from build123d import *

# Parameters (mm, degrees)
ESQUISSE1_R                  = 23
BOSS_EXTRU_1_DEPTH           = 6
ESQUISSE2_R                  = 12.5
BOSS_EXTRU_2_DEPTH           = 10
ESQUISSE3_R                  = 3.25
ENL_V_MAT_EXTRU_1_DEPTH      = 16
ENL_V_MAT_EXTRU_2_REACH      = 38.249
ENL_V_MAT_EXTRU_2_END_RADIUS = 12.5
ESQUISSE4_R                  = 2.5
ESQUISSE5_R                  = 2.75
ENL_V_MAT_EXTRU_3_DEPTH      = 6
R_P_T_PAR_COURBE1_COUNT      = 3
ENL_V_MAT_EXTRU_4_REACH      = 38.249
ESQUISSE6_W                  = 8
ESQUISSE6_H                  = 4


with BuildPart() as part:
    # Esquisse1 → Boss.-Extru.1 (new body)
    with BuildSketch(Plane.XY):
        Circle(ESQUISSE1_R)
    extrude(amount=BOSS_EXTRU_1_DEPTH)

    # Esquisse2 → Boss.-Extru.2 (add)
    with BuildSketch(Plane.XY.offset(6)):
        Circle(ESQUISSE2_R)
    extrude(amount=BOSS_EXTRU_2_DEPTH)

    # Esquisse3 → Enlèv. mat.-Extru.1 (cut)
    with BuildSketch(Plane.XY.offset(16)):
        Circle(ESQUISSE3_R)
    extrude(amount=-ENL_V_MAT_EXTRU_1_DEPTH, mode=Mode.SUBTRACT)

    # Enlèv. mat.-Extru.2: up to this cylinder (the profile starts inside it)
    enl_v_mat_extru_2_end = Plane(origin=(0, 0, 11), z_dir=(0, 0, -1)) * Cylinder(ENL_V_MAT_EXTRU_2_END_RADIUS, 102.498, mode=Mode.PRIVATE)
    # Esquisse4 → Enlèv. mat.-Extru.2 (cut, up to the surface)
    with BuildSketch(Plane(origin=(0, 0, 0), x_dir=(1, 0, 0), z_dir=(0, 1, 0)), mode=Mode.PRIVATE) as enl_v_mat_extru_2_sk1:
        with Locations(Location((0, -11, 0), (0, 0, 270))):
            Circle(ESQUISSE4_R)
    enl_v_mat_extru_2_tool1 = extrude(enl_v_mat_extru_2_sk1.sketch, amount=-ENL_V_MAT_EXTRU_2_REACH, mode=Mode.PRIVATE) & enl_v_mat_extru_2_end
    add(enl_v_mat_extru_2_tool1.solids().sort_by_distance((0, 0, 11))[0], mode=Mode.SUBTRACT)

    # Esquisse5 → Enlèv. mat.-Extru.3 (cut)
    with BuildSketch(Plane.XY.offset(6)):
        with Locations((0, 18)):
            Circle(ESQUISSE5_R)
    enl_v_mat_extru_3 = extrude(amount=-ENL_V_MAT_EXTRU_3_DEPTH, mode=Mode.SUBTRACT)

    # Répét. par courbe1: Enlèv. mat.-Extru.3 ×3 about axis
    r_p_t_par_courbe1_axis = Axis((0, 0, 6), (0, 0, -1))
    for i in range(1, R_P_T_PAR_COURBE1_COUNT):
        add(enl_v_mat_extru_3.rotate(r_p_t_par_courbe1_axis, i * 360 / R_P_T_PAR_COURBE1_COUNT), mode=Mode.SUBTRACT)

    # Enlèv. mat.-Extru.4: up to this face of the body (flat: up to its plane)
    enl_v_mat_extru_4_end = Plane(part.part.faces().sort_by_distance((-22.349461761, 0, 6))[0])
    # Esquisse6 → Enlèv. mat.-Extru.4 (cut, up to the picked face)
    with BuildSketch(Plane.XY.offset(16), mode=Mode.PRIVATE) as enl_v_mat_extru_4_sk1:
        with Locations((0, -7)):
            Rectangle(ESQUISSE6_W, ESQUISSE6_H)
    enl_v_mat_extru_4_tool1 = split(extrude(enl_v_mat_extru_4_sk1.sketch, amount=-ENL_V_MAT_EXTRU_4_REACH, mode=Mode.PRIVATE), bisect_by=enl_v_mat_extru_4_end, keep=Keep.BOTH, mode=Mode.PRIVATE)
    add(enl_v_mat_extru_4_tool1.solids().sort_by(Axis((0, -7, 16), (0, 0, -1)))[0], mode=Mode.SUBTRACT)


solid = part.part
Part model, mm, in its own coordinate system. A direction names the side the tool comes from. Give positions to 0.01 mm unless a question says otherwise; leave off trailing zeros. Loops run counter-clockwise (first coordinate to the right, second up) from the corner with the lowest first, then second, coordinate; pieces in that order, holes last.
(1) Band-saw the part on D-D (y = -4). Write the cut outline in (x, z).
Return value:
outline: (-22.65, 0) - (22.65, 0) - (22.65, 6) - (11.84, 6) - (11.84, 16) - (-11.84, 16) - (-11.84, 6) - (-22.65, 6) - close; hole circle Ø5 at (0, 11)
(2) Pull direction Y, two halves, no side cores. Call faces 1 (the cylindrical face through (11.923, 3.755, 10.93)), 2 (the flat face through (3, 3, 16)), 3 (the cylindrical face through (18.13, -10.05, 3.04)): pulls with the +Y half, pulls with the -Y half, needs draft (parallel to the pull), parting line crosses it, or undercut.
Return value:
face 1: parting line crosses it
face 2: needs draft
face 3: undercut
(3) Band-saw the part on A-A (x = 0). Write the cut outline in (y, z), and give its area (3 significant figures).
Return value:
outline: (-23, 0) - (-3.25, 0) - (-3.25, 8.5) - (-5, 8.5) - (-5, 6) - (-9, 6) - (-9, 8.5) - (-12.5, 8.5) - (-12.5, 6) - (-23, 6) - close; (-12.5, 13.5) - (-9, 13.5) - (-9, 16) - (-12.5, 16) - close; (-5, 13.5) - (-3.25, 13.5) - (-3.25, 16) - (-5, 16) - close; (3.25, 0) - (15.25, 0) - (15.25, 6) - (12.5, 6) - (12.5, 16) - (3.25, 16) - close; (20.75, 0) - (23, 0) - (23, 6) - (20.75, 6) - close
area: 323 mm2
(4) Pin check, flat tips, straight feed: pin 1 (4 mm diameter, centred on y = 6, z = 4.5, fed in from -X); pin 2 (2 mm diameter, centred on x = 0.5, y = -7, fed in from +Z); pin 3 (8 mm diameter, centred on x = 8, z = 10.5, fed in from -Y). Stop position of each tip, or through.
Return value:
pin 1: stops at x = -22.65
pin 2: stops at z = 6
pin 3: stops at y = -11.84
(5) Band-saw the part on B-B (y = 18). Write the cut outline in (x, z).
Return value:
outline: (-14.32, 0) - (-2.75, 0) - (-2.75, 6) - (-14.32, 6) - close; (2.75, 0) - (14.32, 0) - (14.32, 6) - (2.75, 6) - close
(6) Band-saw the part on C-C (x = -15.5). Write the cut outline in (y, z), and give its area (3 significant figures).
Return value:
outline: (-16.99, 0) - (-11.75, 0) - (-11.75, 6) - (-16.99, 6) - close; (-6.25, 0) - (16.99, 0) - (16.99, 6) - (-6.25, 6) - close
area: 171 mm2
(7) Drill centre lines: line 1 along Y through (x, z) = (0, 2.6); line 2 along Z through (x, y) = (0, -4.15); line 3 along Z through (x, y) = (11, -16.5). Where is each one in solid material? Low to high.
Return value:
line 1: y = -23 to -3.25, 3.25 to 15.25, 20.75 to 23
line 2: z = 0 to 8.5, 13.5 to 16
line 3: z = 0 to 6
(8) 3-axis set-ups, long thin cutter, end or side, ignore diameter. For faces 4 (the cylindrical face through (-0.423, 3.222, 8.112)), 5 (the cylindrical face through (0.751, -3.843, 13.385)), 6 (the flat face through (-4, -7, 11)): which of +Z, -Z, +X, -X, +Y, -Y reach the whole face in a straight line?
Return value:
face 4: +Z, -Z
face 5: -Y
face 6: +Z
